Work out the finished part from the listing and answer in its coordinate system (mm). Coordinates: 2 decimals unless noted, no trailing zeros. Order: outer loops, then holes, each group sorted by start corner. A loop starts at its lowest first (then second) coordinate and runs counter-clockwise, first axis right, second up. Notation, with made-up numbers: (67, -31) -> (78, -31) arc R14 cw to (78, -9) -> close; hole circle Ø4 at (44, 15). An arc over 180 degrees is marked (long way). Answer as CSV lines item,"result". Start each with the question number.
Item 1: Straight lines are drawn through the part: L1, parallel to X at y = -4, z = 0.35; L2, parallel to Z at x = 4.25, y = -7; L3, parallel to X at y = -2.75, z = 0.25. For each, find the intervals that lie inside material, in ascending order.
Item 2: Section A-A (y = -1.5) is taken. Write down the section's boundary in (x, z), then the cut area to 3 significant figures.
Item 3: For a pull along X with two mould halves and no side action, classify faces 1 (the face through (2, -5, 0.5)), 2 (the face through (6.75, -4.48, 0.78)), 3 (the face through (12.98, -6.18, 2.04)), 4 (the face through (18.987, -5.07, 2.085)) as pulls with the +X half, pulls with the -X half, needs draft (parallel to the pull), parting line crosses it, or undercut.
Item 4: Section C-C (x = 17.5) is taken. Write down the section's boundary in (y, z).
Item 5: Each of these flat-tipped pins is pushed along its axis until it touches: pin 1 Ø5 at (x, y) = (17, -3) entering from -Z; pin 2 Ø4 at (x, y) = (10.5, -4) entering from -Z; pin 3 Ø4.5 at (x, y) = (2, -5.5) entering from +Z; pin 4 Ø0.6 at (y, z) = (-6.5, 0) entering from +X. Where does it stop, or does it pass through?
Item 6: Section B-B (x = 22.75) is taken. Write down the section's boundary in (y, z).
```python
from build123d import *

# Parameters (mm, degrees)
SKETCH2_W                                         = 10
SKETCH2_H                                         = 10
BOSS_EXTRUDE1_DEPTH                               = 0.5
BOSS_EXTRUDE2_DEPTH                               = 10
CSK_FOR_1_FLAT_HEAD_SOCKET_CAP_SCREW1_D           = 2.0574
CSK_FOR_1_FLAT_HEAD_SOCKET_CAP_SCREW1_CSINK_D     = 4.2672
CSK_FOR_1_FLAT_HEAD_SOCKET_CAP_SCREW1_CSINK_ANGLE = 82
CSK_FOR_1_FLAT_HEAD_SOCKET_CAP_SCREW2_D           = 2.0574
CSK_FOR_1_FLAT_HEAD_SOCKET_CAP_SCREW2_CSINK_D     = 4.2672
CSK_FOR_1_FLAT_HEAD_SOCKET_CAP_SCREW2_CSINK_ANGLE = 82


with BuildPart() as part:
    # Sketch2 → Boss-Extrude1 (new body)
    with BuildSketch(Plane.XY):
        with Locations((5, -5)):
            Rectangle(SKETCH2_W, SKETCH2_H)
    extrude(amount=BOSS_EXTRUDE1_DEPTH)

    # Sketch3 → Boss-Extrude2 (add)
    with BuildSketch(Plane.XZ.offset(10)):
        Polygon((4.241229517, 0.5), (21.967769071, 3.625667198), (27.726539554, 3.625667198), (10, 0.5), align=None)
    extrude(amount=-BOSS_EXTRUDE2_DEPTH)

    # CSK for #1 Flat Head Socket Cap Screw1 (through all)
    with Locations(Plane(origin=(0, 0, 0), x_dir=(-1, 0, 0), z_dir=(0, 0, -1))):
        with Locations((-5.362516401, -4.921292394)):
            CounterSinkHole(CSK_FOR_1_FLAT_HEAD_SOCKET_CAP_SCREW1_D / 2, CSK_FOR_1_FLAT_HEAD_SOCKET_CAP_SCREW1_CSINK_D / 2, counter_sink_angle=CSK_FOR_1_FLAT_HEAD_SOCKET_CAP_SCREW1_CSINK_ANGLE)

    # CSK for #1 Flat Head Socket Cap Screw2 (through all)
    with Locations(Plane(origin=(0.21603186, 0, -1.225177561), x_dir=(-0.984807753, 0, -0.173648178), z_dir=(0.173648178, 0, -0.984807753))):
        with Locations((-14.39146791, -4.879407471)):
            CounterSinkHole(CSK_FOR_1_FLAT_HEAD_SOCKET_CAP_SCREW2_D / 2, CSK_FOR_1_FLAT_HEAD_SOCKET_CAP_SCREW2_CSINK_D / 2, counter_sink_angle=CSK_FOR_1_FLAT_HEAD_SOCKET_CAP_SCREW2_CSINK_ANGLE)


solid = part.part
```
Checked values:
1,L1,"x = 0 to 3.78, 6.94 to 10"
1,L2,"z = 0 to 0.5"
1,L3,"x = 0 to 10"
2,outline,"(0, 0) -> (10, 0) -> (10, 0.5) -> (27.73, 3.63) -> (21.97, 3.63) -> (4.24, 0.5) -> (0, 0.5) -> close"
2,area,"23.0 mm^2"
3,face 1,"needs draft"
3,face 2,"undercut"
3,face 3,"pulls with the -X half"
3,face 4,"pulls with the +X half"
4,outline,"(-10, 1.82) -> (0, 1.82) -> (0, 2.84) -> (-10, 2.84) -> close"
5,pin 1,"stops at z = 1.3"
5,pin 2,"stops at z = 0"
5,pin 3,"stops at z = 0.5"
5,pin 4,"stops at x = 10"
6,outline,"(-10, 2.75) -> (0, 2.75) -> (0, 3.63) -> (-10, 3.63) -> close"
